Answer from the drawing. Dimensions are ordinates in mm from the lowest x, y and z of the part. Round coordinates to 2 decimals unless told otherwise and drop trailing zeros. Write each loop counter-clockwise with the first axis right and the second up, starting at its lowest first coordinate (ties: lowest second). Pieces come first, ordered by that corner, then holes. Notation, with made-up numbers: (21, 24) - (48, 24) arc R11 ccw to (48, 44) - close; hole circle Ø2 at (-22, -27.5). An arc over 180 degrees is marked (long way). Answer as CSV lines item,"result". Start each with the question number.
1) Find section B-B on y = 12. Determine the outline of the cut face in (x, z).
2) Find section C-C on z = 9. Determine the outline of the cut face in (x, y).
3) Find section A-A on x = 23. Determine the outline of the cut face in (y, z).
4) Each of these flat-tipped pins is pushed along its axis until it touches: pin 1 (2 mm diameter, centred on x = 11, z = 15, fed in from +Y); pin 2 (1.8 mm diameter, centred on y = 12, z = 9, fed in from +X); pin 3 (3 mm diameter, centred on x = 24, z = 10.5, fed in from -Y); pin 4 (3.5 mm diameter, centred on x = 23, y = 12, fed in from -Z). Where does it stop, or does it pass through?
5) Consider line 1 along Z through (x, y) = (26.05, 12); line 2 along Y through (x, z) = (23, 7.5); line 3 along Y through (x, z) = (25.85, 9). Determine where each line is inside the solid, lowest interval first.
6) For a pull along Y with two mould halves and no side action, classify the marked faces 1, 2 and 3 as +Y half, -Y half, draft (parallel to the pull), parting line (faces both ways), or undercut.
7) Find section D-D on x = 26. Determine the outline of the cut face in (y, z), then the cut area to 3 significant figures.
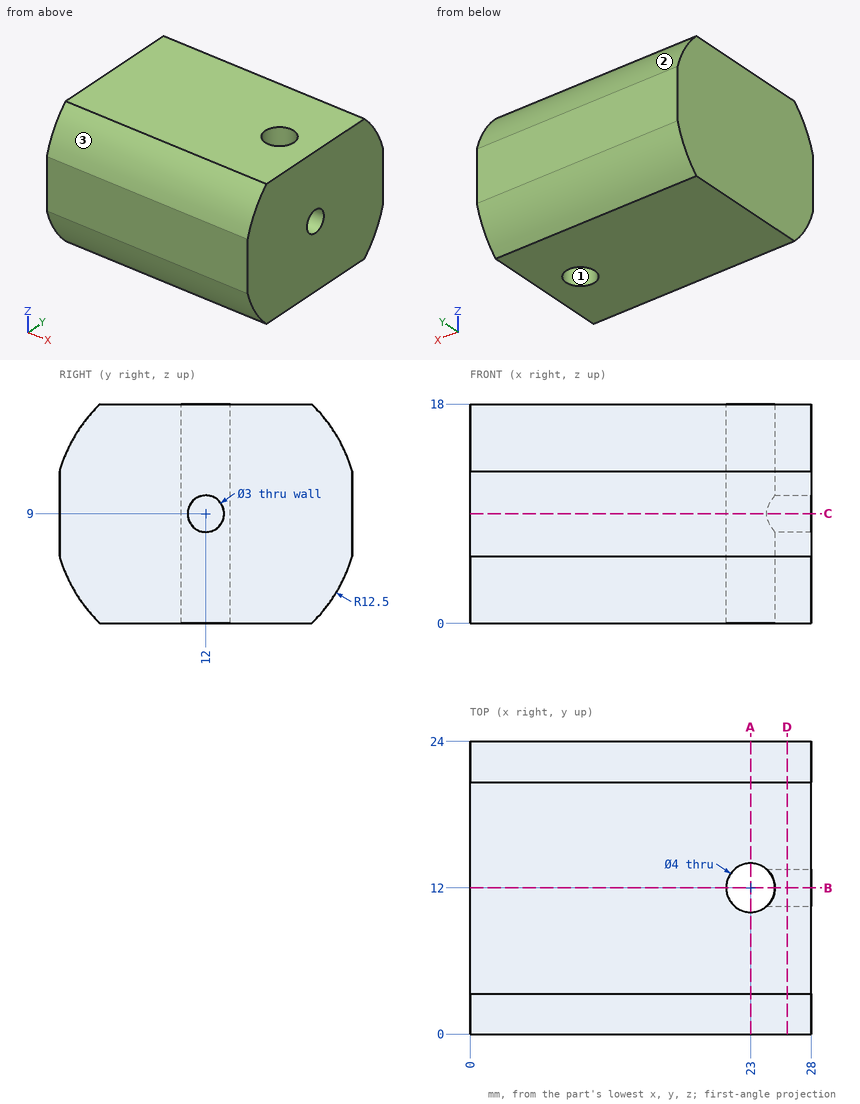
Check values:
1,outline,"(0, 0) - (21, 0) - (21, 18) - (0, 18) - close; (25, 0) - (28, 0) - (28, 7.5) - (25, 7.5) - close; (25, 10.5) - (28, 10.5) - (28, 18) - (25, 18) - close"
2,outline,"(0, 0) - (28, 0) - (28, 10.5) - (24.32, 10.5) arc R2 cw (long way) to (24.32, 13.5) - (28, 13.5) - (28, 24) - (0, 24) - close"
3,outline,"(0, 5.5) arc R12.5 ccw to (3.33, 0) - (10, 0) - (10, 18) - (3.33, 18) arc R12.5 ccw to (0, 12.5) - close; (14, 0) - (20.67, 0) arc R12.5 ccw to (24, 5.5) - (24, 12.5) arc R12.5 ccw to (20.67, 18) - (14, 18) - close"
4,pin 1,"stops at y = 23.46"
4,pin 2,"stops at x = 21.21"
4,pin 3,"stops at y = 0"
4,pin 4,"passes through"
5,line 1,"z = 0 to 7.5, 10.5 to 18"
5,line 2,"y = 0 to 10, 14 to 24"
5,line 3,"y = 0 to 10.5, 13.5 to 24"
6,face 1,"undercut"
6,face 2,"+Y half"
6,face 3,"-Y half"
7,outline,"(0, 5.5) arc R12.5 ccw to (3.33, 0) - (20.67, 0) arc R12.5 ccw to (24, 5.5) - (24, 12.5) arc R12.5 ccw to (20.67, 18) - (3.33, 18) arc R12.5 ccw to (0, 12.5) - close; hole circle Ø3 at (12, 9)"
7,area,"396 mm^2"
